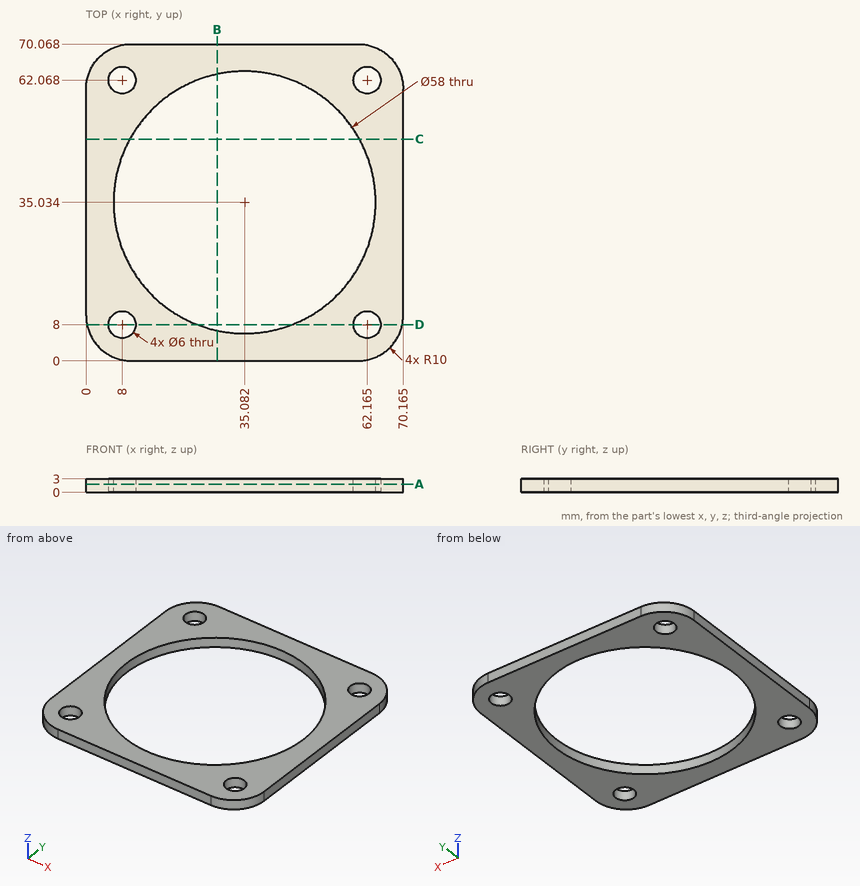
Design review of the part shown in the three views and the two pictorial views. Dimensions are in mm from the part's minimum x, y and z. Coordinates: 2 decimals unless noted, no trailing zeros. Loops run counter-clockwise (first coordinate to the right, second up) from the corner with the lowest first, then second, coordinate; pieces in that order, holes last. Notation, with made-up numbers: M 33,41.25 L 89,41.25 A14 ccw 89,65.25 Z; hole C 60.5,-34 d10. An arc over 180 degrees is marked long. Put each result on its own line as item: value. Start each with the question number.
Q1. Wall thickness on line 1 (Y direction, x = 60, z = 2.15) (1 decimal); line 2 (Y direction, x = 36, z = 0.6); line 3 (Y direction, x = 61, z = 0.55) (1 decimal): over which ranges is each line inside the solid? List them lowest first.
Q2. Add section A-A (z = 1.8). Write out the cut boundary in (x, y) (1 decimal).
Q3. Add section D-D (y = 8). Write out the cut boundary in (x, z) (1 decimal).
Q4. Add section B-B (x = 29). Write out the cut boundary in (y, z).
Q5. Clearance check with flat-ended pins moving along their axes: pin 1 (12 mm diameter, centred on x = 19, y = 27.5, fed in from +Z); pin 2 (7 mm diameter, centred on x = 62.16, y = 8, fed in from +Z). State where each tip first meets the part, or that it passes through.
Q6. Add section C-C (y = 49). Write out the cut boundary in (x, z) (1 decimal), and give its area (3 significant figures).
Answers:
1. line 1: y = 0 to 5.9, 10.1 to 20.2, 49.9 to 60, 64.1 to 70.1
1. line 2: y = 0 to 6.05, 64.02 to 70.07
1. line 3: y = 0 to 5.2, 10.8 to 22, 48 to 59.3, 64.8 to 70
2. outline: M 0,10 A10 ccw 10,0 L 60.2,0 A10 ccw 70.2,10 L 70.2,60.1 A10 ccw 60.2,70.1 L 10,70.1 A10 ccw 0,60.1 Z; hole C 8,8 d6; hole C 8,62.1 d6; hole C 35.1,35 d58; hole C 62.2,8 d6; hole C 62.2,62.1 d6
3. outline: M 0.2,0 L 5,0 L 5,3 L 0.2,3 Z; M 11,0 L 24.6,0 L 24.6,3 L 11,3 Z; M 45.6,0 L 59.2,0 L 59.2,3 L 45.6,3 Z; M 65.2,0 L 70,0 L 70,3 L 65.2,3 Z
4. outline: M 0,0 L 6.68,0 L 6.68,3 L 0,3 Z; M 63.39,0 L 70.07,0 L 70.07,3 L 63.39,3 Z
5. pin 1: passes through
5. pin 2: stops at z = 3
6. outline: M 0,0 L 9.7,0 L 9.7,3 L 0,3 Z; M 60.5,0 L 70.2,0 L 70.2,3 L 60.5,3 Z
6. area: 58.0 mm^2
